Source: CAD feature listing. Evaluate the final solid. Frame: model axes, mm. A direction names the side the tool comes from. Round coordinates to 2 decimals unless told otherwise and drop trailing zeros. Order: outer loops, then holes, each group sorted by start corner. A loop starts at its lowest first (then second) coordinate and runs counter-clockwise, first axis right, second up. Notation, with made-up numbers: M -20,46 L 29,46 A35 ccw 29,79 Z; hole C 14.25,23 d3. An arc over 180 degrees is marked long. Use one line per item in the form item = value. Start each with the question number.
Q1. Section D-D (x = -17). Return the cut outline in (y, z).
Q2. Section C-C (y = 32). Return the cut outline in (x, z), plus the area to 3 significant figures.
Q3. Section B-B (x = 0). Return the cut outline in (y, z).
Q4. Pull-direction query (X, two-part tool) for faces 1 (the flat face through (0, 0, 50)), 2 (the cylindrical face through (-5.5, -24.9, 72.2)), 3 (the flat face through (-50, -1, -1)), 4 (the flat face through (-1, -1, -50)); classes: pulls with the +X half, pulls with the -X half, needs draft (parallel to the pull), parting line crosses it, or undercut.
Q5. Contact query for flat-ended pins moving along their axis: pin 1 (4 mm diameter, centred on x = -28, z = 79.5, fed in from +Y); pin 2 (10 mm diameter, centred on x = 3, y = 39, fed in from +Z); pin 3 (2 mm diameter, centred on x = -13, z = 69, fed in from -Y). Output: stop coordinate, or through.
Q6. Section A-A (z = 0). Return the cut outline in (x, y).
Q7. Material intervals for probe 1 along Z at (x, y) = (0, 19); probe 2 along Y at (x, z) = (0, 74); probe 3 along Z at (x, y) = (-1, -29), sorted ascending.
Q8. Reachability of faces 5 (the flat face through (50, -1, -1)), 6 (the cylindrical face through (-29.97, 1.32, 72.18)) from +Z, -Z, +X, -X, +Y, -Y: full face, straight path, thin tool, end or side. Return the list, or none.
from build123d import *

# Parameters (mm, degrees)
F0_W     = 100
F0_H     = 100
F0_R     = 25.5
F1_DEPTH = 50
F2_R     = 30
F2_R_2   = 25.5
F3_DEPTH = 45


with BuildPart() as f1:
    # F0 (on Front) → F1 (new body, symmetric)
    with BuildSketch(Plane.XZ):
        Rectangle(F0_W, F0_H)
        Circle(F0_R, mode=Mode.SUBTRACT)
    extrude(amount=F1_DEPTH, both=True)

    # F2 (on face) → F3 (join)
    with BuildSketch(Plane.XY.offset(50)):
        Circle(F2_R)
        Circle(F2_R_2, mode=Mode.SUBTRACT)
    extrude(amount=F3_DEPTH)


solid = f1.part
Results list:
q1.outline = M -50,-50 L 50,-50 L 50,-19.01 L -50,-19.01 Z; M -50,19.01 L 50,19.01 L 50,50 L 24.72,50 L 24.72,95 L 19.01,95 L 19.01,50 L -19.01,50 L -19.01,95 L -24.72,95 L -24.72,50 L -50,50 Z
q2.outline = M -50,-50 L 50,-50 L 50,50 L -50,50 Z; hole C 0,0 d51
q2.area = 7,960 mm2
q3.outline = M -50,-50 L 50,-50 L 50,-25.5 L -50,-25.5 Z; M -50,25.5 L 50,25.5 L 50,50 L 30,50 L 30,95 L 25.5,95 L 25.5,50 L -25.5,50 L -25.5,95 L -30,95 L -30,50 L -50,50 Z
q4.face_1 = undercut
q4.face_2 = undercut
q4.face_3 = pulls with the -X half
q4.face_4 = needs draft
q5.pin_1 = 14.97
q5.pin_2 = 50
q5.pin_3 = -27.5
q6.outline = M -50,-50 L -25.5,-50 L -25.5,50 L -50,50 Z; M 25.5,-50 L 50,-50 L 50,50 L 25.5,50 Z
q7.probe_1 = -50 to -25.5, 25.5 to 50
q7.probe_2 = -30 to -25.5, 25.5 to 30
q7.probe_3 = -50 to -25.48, 25.48 to 95
q8.face_5 = +Z, -Z, +X, +Y, -Y
q8.face_6 = +Z
